```python
from build123d import *

# Parameters (mm, degrees)
SKETCH1_W           = 180
SKETCH1_H           = 110
SKETCH1_R           = 42
SKETCH1_R_2         = 18.1
BOSS_EXTRUDE1_DEPTH = 6
SKETCH3_R           = 0.5
CUT_EXTRUDE1_DEPTH  = 30


with BuildPart() as part:
    # Sketch1 → Boss-Extrude1 (new body)
    with BuildSketch(Plane.XY):
        with Locations((90, 55)):
            Rectangle(SKETCH1_W, SKETCH1_H)
        with Locations((60, 50)):
            Circle(SKETCH1_R, mode=Mode.SUBTRACT)
        with Locations((140, 60)):
            Circle(SKETCH1_R_2, mode=Mode.SUBTRACT)
    extrude(amount=BOSS_EXTRUDE1_DEPTH)

    # Sketch3 → Cut-Extrude1 (cut)
    with BuildSketch(Plane.XY):
        with Locations((92.880465325, 82.880465325)):
            Circle(SKETCH3_R)
        with Locations((27.119534675, 82.880465325)):
            Circle(SKETCH3_R)
        with Locations((27.119534675, 17.119534675)):
            Circle(SKETCH3_R)
        with Locations((92.880465325, 17.119534675)):
            Circle(SKETCH3_R)
        with Locations((155.202795796, 75.202795796)):
            Circle(SKETCH3_R)
        with Locations((124.797204204, 75.202795796)):
            Circle(SKETCH3_R)
        with Locations((124.797204204, 44.797204204)):
            Circle(SKETCH3_R)
        with Locations((155.202795796, 44.797204204)):
            Circle(SKETCH3_R)
    extrude(amount=CUT_EXTRUDE1_DEPTH, mode=Mode.SUBTRACT)


solid = part.part
```
Could you check a few things on this model? Use its own coordinates, in mm. Give positions to 0.01 mm unless a question says otherwise; leave off trailing zeros. Loops run counter-clockwise (first coordinate to the right, second up) from the corner with the lowest first, then second, coordinate; pieces in that order, holes last. Notation, with made-up numbers: (59, 45.5) - (92, 45.5) arc R7 ccw to (92, 54.5) - close; hole circle Ø8 at (-1, 35.25). An arc over 180 degrees is marked (long way). Use one line per item in the form item = value.
1. I want a section at C-C (y = 33). Please give me the cut outline in (x, z), and give its area (3 significant figures).
Response values:
outline = (0, 0) - (21.59, 0) - (21.59, 6) - (0, 6) - close; (98.41, 0) - (180, 0) - (180, 6) - (98.41, 6) - close
area = 619 mm²
2. I want a section at B-B (y = 50). Please give me the cut outline in (x, z).
Response values:
outline = (0, 0) - (18, 0) - (18, 6) - (0, 6) - close; (102, 0) - (124.91, 0) - (124.91, 6) - (102, 6) - close; (155.09, 0) - (180, 0) - (180, 6) - (155.09, 6) - close
3. I need wall thicknesses on probe 1 along X at (y, z) = (64, 2.3); probe 2 along X at (y, z) = (48, 3.7); probe 3 along Y at (x, z) = (140, 3). Which ranges of each line are inside material? Lowest first, please.
Response values:
probe_1 = 0 to 20.4, 99.6 to 122.35, 157.65 to 180
probe_2 = 0 to 18.05, 101.95 to 126.45, 153.55 to 180
probe_3 = 0 to 41.9, 78.1 to 110
4. I want a section at A-A (x = 140). Please give me the cut outline in (y, z).
Response values:
outline = (0, 0) - (41.9, 0) - (41.9, 6) - (0, 6) - close; (78.1, 0) - (110, 0) - (110, 6) - (78.1, 6) - close
5. I want a section at D-D (z = 3.5). Give the number of separate pieces and of enclosed holes in the cut face, and give its area (3 significant figures).
Response values:
separate_pieces = 1
enclosed_holes = 10
area = 13,200 mm²
6. Thinking about a two-plate mould opening in Y: for faces 1 (the face through (0, 54, 3)), 2 (the face through (137.644, 77.946, 2.958)), 3 (the face through (89, 0, 3)), which applies, released by +Y, released by -Y, zero draft, split by the parting line, or undercut?
Response values:
face_1 = zero draft
face_2 = undercut
face_3 = released by -Y
